Source: three-view drawing plus pictorial views. Frame: mm from the lowest corner of the part. A direction names the side the tool comes from. Coordinates: 2 decimals unless noted, no trailing zeros. Order: outer loops, then holes, each group sorted by start corner. A loop starts at its lowest first (then second) coordinate and runs counter-clockwise, first axis right, second up. Notation, with made-up numbers: (-4, 25.5) -> (32, 25.5) arc R30 cw to (32, 50.5) -> close; hole circle Ø11 at (73.5, 25). An arc over 180 degrees is marked (long way). Use one line per item in the form item = value. Start each with the question number.
1) Access query for the marked faces 1, 2 and 3. Directions: +Z, -Z, +X, -X, +Y, -Y. A direction counts if a zero-diameter tool reaches every point of the face in a straight line with its end or side. Return the directions, or none.
2) Section query D-D on x = 3.25. Output: boundary loops of the cut face in (y, z).
3) Section query B-B on x = 13.2. Output: boundary loops of the cut face in (y, z) (3 decimals), then the cut area to 3 significant figures.
4) Pin query (flat end, axial travel): pin 1 (1 mm diameter, centred on y = 5, z = 0.5, fed in from -X); pin 2 (1 mm diameter, centred on x = 1, z = 1, fed in from +Y); pin 3 (0.6 mm diameter, centred on y = 5.5, z = 0.5, fed in from +X). Return the tip coordinate at first contact, or that it passes through.
5) Draft query along X for the marked faces 4, 5 and 6. Return one class per face: pulls with the +X half, pulls with the -X half, needs draft (parallel to the pull), parting line crosses it, or undercut.
6) Section query C-C on z = 0.3. Output: boundary loops of the cut face in (x, y) (3 decimals).
7) Section query A-A on y = 8. Output: boundary loops of the cut face in (x, z).
8) Ray query, line 1 along Y through (x, z) = (2.75, 1.5); line 2 along Y through (x, z) = (13.75, 1); line 3 along Y through (x, z) = (3, 1.4) (3 decimals). Return the intervals inside material, ascending.
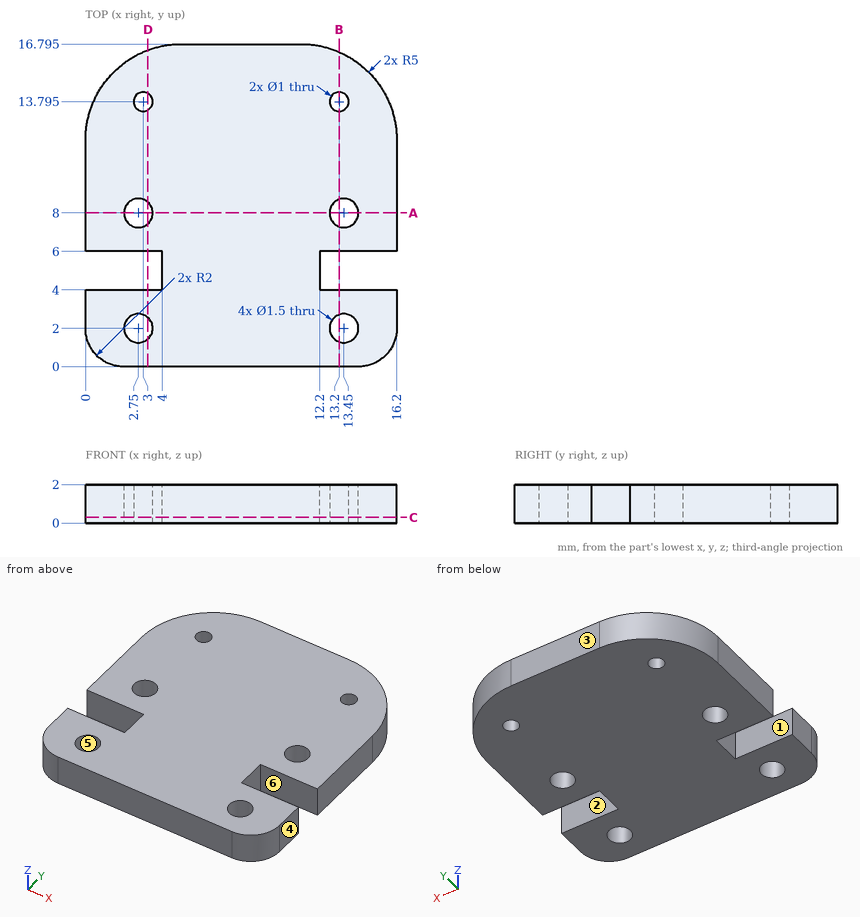
Answers below:
q1.face_1 = +Z, -Z, -X
q1.face_2 = +Z, -Z, +X
q1.face_3 = +Z, -Z, +X, -X, +Y
q2.outline = (0, 0) -> (1.44, 0) -> (1.44, 2) -> (0, 2) -> close; (2.56, 0) -> (4, 0) -> (4, 2) -> (2.56, 2) -> close; (6, 0) -> (7.44, 0) -> (7.44, 2) -> (6, 2) -> close; (8.56, 0) -> (13.36, 0) -> (13.36, 2) -> (8.56, 2) -> close; (14.23, 0) -> (16.48, 0) -> (16.48, 2) -> (14.23, 2) -> close
q3.outline = (0, 0) -> (1.293, 0) -> (1.293, 2) -> (0, 2) -> close; (2.707, 0) -> (4, 0) -> (4, 2) -> (2.707, 2) -> close; (6, 0) -> (7.293, 0) -> (7.293, 2) -> (6, 2) -> close; (8.707, 0) -> (13.295, 0) -> (13.295, 2) -> (8.707, 2) -> close; (14.295, 0) -> (16.378, 0) -> (16.378, 2) -> (14.295, 2) -> close
q3.area = 21.1 mm^2
q4.pin_1 = 4
q4.pin_2 = 15.37
q4.pin_3 = 12.2
q5.face_4 = pulls with the +X half
q5.face_5 = undercut
q5.face_6 = needs draft
q6.outline = (0, 2) arc R2 ccw to (2, 0) -> (14.2, 0) arc R2 ccw to (16.2, 2) -> (16.2, 4) -> (12.2, 4) -> (12.2, 6) -> (16.2, 6) -> (16.2, 11.795) arc R5 ccw to (11.2, 16.795) -> (5, 16.795) arc R5 ccw to (0, 11.795) -> (0, 6) -> (4, 6) -> (4, 4) -> (0, 4) -> close; hole circle Ø1.5 at (2.75, 2); hole circle Ø1.5 at (2.75, 8); hole circle Ø1 at (3, 13.795); hole circle Ø1.5 at (13.45, 2); hole circle Ø1.5 at (13.45, 8); hole circle Ø1 at (13.2, 13.795)
q7.outline = (0, 0) -> (2, 0) -> (2, 2) -> (0, 2) -> close; (3.5, 0) -> (12.7, 0) -> (12.7, 2) -> (3.5, 2) -> close; (14.2, 0) -> (16.2, 0) -> (16.2, 2) -> (14.2, 2) -> close
q8.line_1 = 0 to 1.25, 2.75 to 4, 6 to 7.25, 8.75 to 13.36, 14.23 to 16.26
q8.line_2 = 0 to 1.31, 2.69 to 4, 6 to 7.31, 8.69 to 16.1
q8.line_3 = 0 to 1.293, 2.707 to 4, 6 to 7.293, 8.707 to 13.295, 14.295 to 16.378
